```python
from build123d import *

# Parameters (mm, degrees)
EXTRUDE_1_DEPTH     = 25
SKETCH_2_R          = 1.5
CUT_EXTRUDE_1_DEPTH = 5


with BuildPart() as part:
    # 草图1 → 凸台-拉伸1 (new body)
    with BuildSketch(Plane.XY):
        with BuildLine():
            Line((0, 12.5), (65, 12.5))
            ThreePointArc((65, 12.5), (77.5, 0), (65, -12.5))
            Line((65, -12.5), (0, -12.5))
            ThreePointArc((0, -12.5), (-12.5, 0), (0, 12.5))
        make_face()
    extrude(amount=EXTRUDE_1_DEPTH)

    # 草图2 → 切除-拉伸1 (cut)
    with BuildSketch(Plane(origin=(0, 0, 0), x_dir=(-1, 0, 0), z_dir=(0, 0, -1))):
        with Locations((-9.75, 0)):
            Circle(SKETCH_2_R)
        with Locations(Location((-55.25, 0, 0), (0, 0, 180))):
            Circle(SKETCH_2_R)
    extrude(amount=-CUT_EXTRUDE_1_DEPTH, mode=Mode.SUBTRACT)


solid = part.part
```
Model file for the job. Use its own axes, mm. A direction names the side the tool comes from. Coordinates: 2 decimals unless noted, no trailing zeros. Loops run counter-clockwise (first coordinate to the right, second up) from the corner with the lowest first, then second, coordinate; pieces in that order, holes last. Notation, with made-up numbers: (27.5, 7) -> (78.5, 7) arc R18 cw to (78.5, 17) -> close; hole circle Ø4 at (71, -31.75). An arc over 180 degrees is marked (long way). Answer as a JSON object with one key per item and string values.
Q1. Pull direction Y, two halves, no side cores. Call faces 1 (the flat face through (33, 0, 0)), 2 (the cylindrical face through (56.68, -0.45, 2.46)), 3 (the flat face through (33, -12.5, 12)), 4 (the cylindrical face through (77.497, 0.275, 12.325)): released by +Y, released by -Y, zero draft, split by the parting line, or undercut.
Report:
{"face 1": "zero draft", "face 2": "undercut", "face 3": "released by -Y", "face 4": "split by the parting line"}
Q2. Cut at C-C (z = 17.75). List the corners of the cut face in (x, y), and give its area (3 significant figures).
Report:
{"outline": "(0, -12.5) -> (65, -12.5) arc R12.5 ccw to (65, 12.5) -> (0, 12.5) arc R12.5 ccw to start", "area": "2,120 mm2"}
Q3. 3-axis set-ups, long thin cutter, end or side, ignore diameter. For faces 5 (the flat face through (33, 0, 25)), 6 (the cylindrical face through (11.25, 0.07, 2.46)): which of +Z, -Z, +X, -X, +Y, -Y reach the whole face in a straight line?
Report:
{"face 5": "+Z, +X, -X, +Y, -Y", "face 6": "-Z"}
Q4. Cut at A-A (x = 55.25). List the corners of the cut face in (y, z), and give its area (3 significant figures).
Report:
{"outline": "(-12.5, 0) -> (-1.5, 0) -> (-1.5, 5) -> (1.5, 5) -> (1.5, 0) -> (12.5, 0) -> (12.5, 25) -> (-12.5, 25) -> close", "area": "610 mm2"}
Q5. Cut at B-B (z = 1.5). List the corners of the cut face in (x, y).
Report:
{"outline": "(0, -12.5) -> (65, -12.5) arc R12.5 ccw to (65, 12.5) -> (0, 12.5) arc R12.5 ccw to start; hole circle Ø3 at (9.75, 0); hole circle Ø3 at (55.25, 0)"}
Q6. Flat gauge pins, fed straight in: P1, Ø4, axis at x = 22, y = 2.5, coming from the -Z side; P2, Ø10, axis at y = -7, z = 12, coming from the +X side; P3, Ø5, axis at y = 5, z = 17, coming from the -X side; P4, Ø1, axis at y = 7.5, z = 3, coming from the +X side. Where does each tip first touch, or does it go through?
Report:
{"P1": "stops at z = 0", "P2": "stops at x = 77.34", "P3": "stops at x = -12.25", "P4": "stops at x = 75.36"}
Q7. Cut at D-D (y = -8.75). List the corners of the cut face in (x, z).
Report:
{"outline": "(-8.93, 0) -> (73.93, 0) -> (73.93, 25) -> (-8.93, 25) -> close"}
Q8. Probe probe 1 along Y at (x, z) = (55.25, 2); probe 2 along X at (y, z) = (-0.25, 18.75); probe 3 along X at (y, z) = (7, 16.25). List the from-to ranges inside material, lowest first.
Report:
{"probe 1": "y = -12.5 to -1.5, 1.5 to 12.5", "probe 2": "x = -12.5 to 77.5", "probe 3": "x = -10.36 to 75.36"}
